Check sheet for the drawn part. Datum: minimum x, y, z corner. Units: mm. A direction names the side the tool comes from. Round coordinates to 2 decimals unless told otherwise and drop trailing zeros. Loops run counter-clockwise (first coordinate to the right, second up) from the corner with the lowest first, then second, coordinate; pieces in that order, holes last.
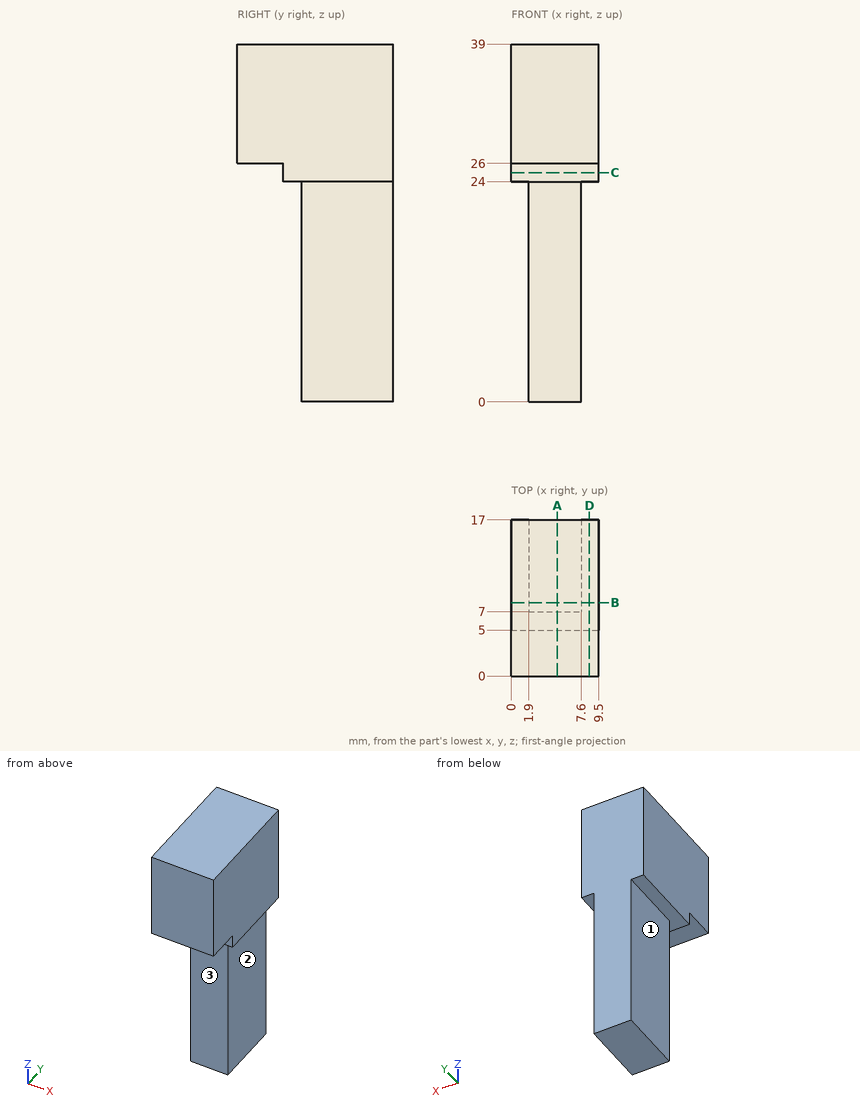
1) Sectioned sample at A-A, the plane x = 5. Record the cut outline in (y, z), then the cut area to 3 significant figures.
Report:
outline: (0, 26) - (5, 26) - (5, 24) - (7, 24) - (7, 0) - (17, 0) - (17, 39) - (0, 39) - close
area: 485 mm2
2) Access from +Z, -Z, +X, -X, +Y, -Y to the whole of each face (thin tool, end or side, straight path). Record for the marked faces 1, 2 and 3.
Report:
face 1: -Z, -X, +Y, -Y
face 2: -Z, +X, +Y, -Y
face 3: -Z, +X, -X, -Y
3) Scan lines: line 1 along X through (y, z) = (10.25, 3); line 2 along Z through (x, y) = (9, 15.75); line 3 along Y through (x, z) = (3.5, 20.5). Record each from-to range of solid material in increasing order.
Report:
line 1: x = 1.9 to 7.6
line 2: z = 24 to 39
line 3: y = 7 to 17
4) Sectioned sample at C-C, the plane z = 25. Record the cut outline in (x, y).
Report:
outline: (0, 5) - (9.5, 5) - (9.5, 17) - (0, 17) - close
5) Gauge pin test, flat ends, axial feed: pin 1 (1.7 mm diameter, centred on x = 5.5, z = 10.5, fed in from -Y); pin 2 (5 mm diameter, centred on y = 13.5, z = 16, fed in from +X); pin 3 (10 mm diameter, centred on y = 4.5, z = 13.5, fed in from -X). Record the tip position at first contact, or that the pin passes through.
Report:
pin 1: stops at y = 7
pin 2: stops at x = 7.6
pin 3: stops at x = 1.9
6) Sectioned sample at D-D, the plane x = 8.5. Record the cut outline in (y, z).
Report:
outline: (0, 26) - (5, 26) - (5, 24) - (17, 24) - (17, 39) - (0, 39) - close
7) Sectioned sample at B-B, the plane y = 8. Record the cut outline in (x, z), then the cut area to 3 significant figures.
Report:
outline: (0, 24) - (1.9, 24) - (1.9, 0) - (7.6, 0) - (7.6, 24) - (9.5, 24) - (9.5, 39) - (0, 39) - close
area: 279 mm2
